Geometry check sheet. Reference: the model listing, model coordinates, mm. Face numbers are marked on the shaded views. Round coordinates to 2 decimals unless told otherwise and drop trailing zeros. Order: outer loops, then holes, each group sorted by start corner. A loop starts at its lowest first (then second) coordinate and runs counter-clockwise, first axis right, second up.
(1) Gauge pin test, flat ends, axial feed: P1, Ø2, axis at x = 19, y = 6, coming from the +Z side; P2, Ø4.5, axis at y = 6, z = 15, coming from the +X side. Record the tip position at first contact, or that the pin passes through.
(2) Cross-section at B-B on x = -18.5. Enter the section's corners in (y, z).
(3) Draft check along Z on the marked faces 1, 2, 3 and 4. Enter one of: pulls with the +Z half, pulls with the -Z half, needs draft (parallel to the pull), parting line crosses it, or undercut.
(4) Cross-section at C-C on z = -11. Enter the section's corners in (x, y), and give its area (3 significant figures).
(5) Thickness scan on L1, parallel to X at y = 1.5, z = -12; L2, parallel to Z at x = 12, y = 1.25. Record the ranges inside material, lowest first.
(6) Cross-section at A-A on y = 7. Enter the section's corners in (x, z).
from build123d import *

# Parameters (mm, degrees)
BOSS_EXTRUDE1_DEPTH = 9.4


with BuildPart() as part:
    # Sketch1 → Boss-Extrude1 (new body)
    with BuildSketch(Plane(origin=(0, 0, 0), x_dir=(1, 0, 0), z_dir=(0, 1, 0))):
        with BuildLine():
            Line((-41.2, -27.4), (-27.066025404, -27.4))
            ThreePointArc((-27.066025404, -27.4), (-26.2, -28.9), (-25.333974596, -27.4))
            Line((-25.333974596, -27.4), (25.333974596, -27.4))
            ThreePointArc((25.333974596, -27.4), (26.2, -28.9), (27.066025404, -27.4))
            Line((27.066025404, -27.4), (41.2, -27.4))
            Line((41.2, -27.4), (41.2, -22.866025404))
            ThreePointArc((41.2, -22.866025404), (42.7, -22), (41.2, -21.133974596))
            Line((41.2, -21.133974596), (41.2, -0.866025404))
            ThreePointArc((41.2, -0.866025404), (42.7, 0), (41.2, 0.866025404))
            Line((41.2, 0.866025404), (41.2, 21.133974596))
            ThreePointArc((41.2, 21.133974596), (42.7, 22), (41.2, 22.866025404))
            Line((41.2, 22.866025404), (41.2, 27.4))
            Line((41.2, 27.4), (-41.2, 27.4))
            Line((-41.2, 27.4), (-41.2, -27.4))
        make_face()
    extrude(amount=BOSS_EXTRUDE1_DEPTH)


solid = part.part
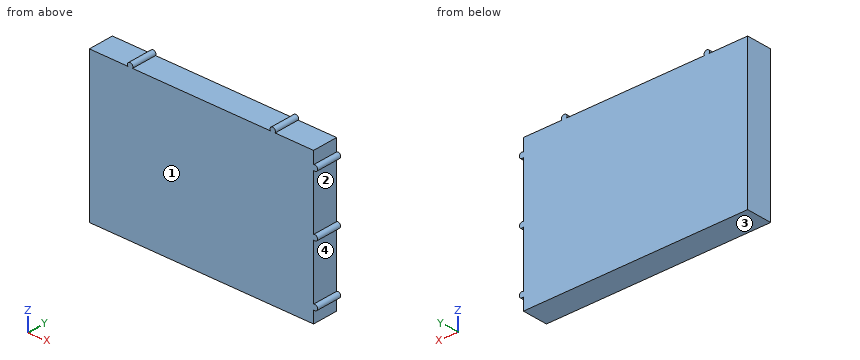
Found:
1. P1: stops at z = 27.4
1. P2: stops at x = 41.2
2. outline: (0, -27.4) - (9.4, -27.4) - (9.4, 27.4) - (0, 27.4) - close
3. face 1: needs draft
3. face 2: undercut
3. face 3: pulls with the -Z half
3. face 4: undercut
4. outline: (-41.2, 0) - (41.2, 0) - (41.2, 9.4) - (-41.2, 9.4) - close
4. area: 775 mm2
5. L1: x = -41.2 to 41.2
5. L2: z = -27.4 to 27.4
6. outline: (-41.2, -27.4) - (41.2, -27.4) - (41.2, -22.87) arc R1 ccw (long way) to (41.2, -21.13) - (41.2, -0.87) arc R1 ccw (long way) to (41.2, 0.87) - (41.2, 21.13) arc R1 ccw (long way) to (41.2, 22.87) - (41.2, 27.4) - (27.07, 27.4) arc R1 ccw (long way) to (25.33, 27.4) - (-25.33, 27.4) arc R1 ccw (long way) to (-27.07, 27.4) - (-41.2, 27.4) - close
